Build history of the part. All positions in model axes, mm. Face numbers are marked on the shaded views. A direction names the side the tool comes from. Give positions to 0.01 mm unless a question says otherwise; leave off trailing zeros. Write each loop counter-clockwise with the first axis right and the second up, starting at its lowest first coordinate (ties: lowest second). Pieces come first, ordered by that corner, then holes. Notation, with made-up numbers: (-36, 18.25) -> (13, 18.25) arc R35 cw to (13, 53.25) -> close; hole circle Ø10 at (50.25, 41). An arc over 180 degrees is marked (long way). Write item = value, one per line. Start each with the question number.
Q1. Mould opens along Y. For the marked faces 1, 2 and 3 say: pulls with the +Y half, pulls with the -Y half, needs draft (parallel to the pull), parting line crosses it, or undercut.
Q2. Saw through at B-B, the plane z = 19.5. List the corners of the cut face in (x, y), then the cut area to 3 significant figures.
Q3. Tool access for the marked faces 4, 5, 6, 7 and 8: list every direction of +Z, -Z, +X, -X, +Y, -Y with a clear straight run to the whole face (end or side of a thin tool).
Q4. Wall check: line 1 (X direction, y = -12, z = -21); line 2 (Y direction, x = 19, z = -1); line 3 (Y direction, x = 28.5, z = 4.5). Give the ranges that are in metal, low to high.
Q5. Drop flat-ended pins along their axis: P1, Ø3, axis at x = 3, y = -22, coming from the +Z side; P2, Ø4, axis at x = 28.5, z = 2, coming from the +Y side; P3, Ø4, axis at x = 23, z = -3, coming from the -Y side. Give the stop position or say it passes through.
Q6. Saw through at C-C, the plane y = -16. List the corners of the cut face in (x, z), then the cut area to 3 significant figures.
Q7. Saw through at D-D, the plane x = 13. List the corners of the cut face in (y, z), then the cut area to 3 significant figures.
Q8. Saw through at A-A, the plane z = 0. List the corners of the cut face in (x, y), then the cut area to 3 significant figures.
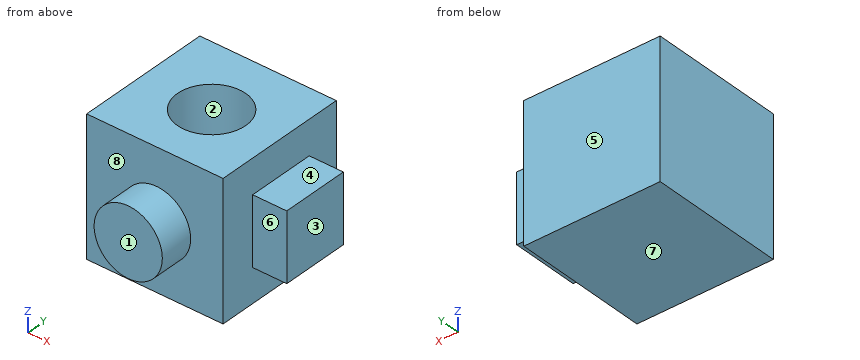
from build123d import *

# Parameters (mm, degrees)
F0_W     = 50.8
F0_H     = 50.8
F1_DEPTH = 50.8
F2_R     = 12.7
F3_DEPTH = 12.7
F4_W     = 25.4
F4_H     = 25.4
F5_DEPTH = 12.7
F6_R     = 12.7
F7_DEPTH = 19.812


with BuildPart() as f1:
    # F0 (on Front) → F1 (new body)
    with BuildSketch(Plane.XZ):
        with Locations((-6.018102, 1.05328)):
            Rectangle(F0_W, F0_H)
    extrude(amount=F1_DEPTH)

    # F2 (on face) → F3 (join)
    with BuildSketch(Plane.XZ.offset(50.8)):
        with Locations((-5.397914, 0)):
            Circle(F2_R)
    extrude(amount=F3_DEPTH)

    # F4 (on face) → F5 (join)
    with BuildSketch(Plane.YZ.offset(19.381898)):
        with Locations((-24.825621, 0.956289)):
            Rectangle(F4_W, F4_H)
    extrude(amount=F5_DEPTH)

    # F6 (on face) → F7 (cut)
    with BuildSketch(Plane.XY.offset(26.45328)):
        with Locations((-5.251253, -26.256265)):
            Circle(F6_R)
    extrude(amount=-F7_DEPTH, mode=Mode.SUBTRACT)


solid = f1.part
Report:
q1.face_1 = pulls with the -Y half
q1.face_2 = undercut
q1.face_3 = needs draft
q2.outline = (-31.42, -50.8) -> (19.38, -50.8) -> (19.38, 0) -> (-31.42, 0) -> close; hole circle Ø25.4 at (-5.25, -26.26)
q2.area = 2,070 mm2
q3.face_4 = +Z, +X, +Y, -Y
q3.face_5 = +Z, -Z, +X, -X, +Y
q3.face_6 = +Z, -Z, +X, -Y
q3.face_7 = -Z, +X, -X, +Y, -Y
q3.face_8 = -Y
q4.line_1 = -31.42 to 19.38
q4.line_2 = -50.8 to 0
q4.line_3 = -37.53 to -12.13
q5.P1 = 6.64
q5.P2 = -12.13
q5.P3 = -37.53
q6.outline = (-31.42, -24.35) -> (19.38, -24.35) -> (19.38, -11.74) -> (32.08, -11.74) -> (32.08, 13.66) -> (19.38, 13.66) -> (19.38, 26.45) -> (2.24, 26.45) -> (2.24, 6.64) -> (-12.74, 6.64) -> (-12.74, 26.45) -> (-31.42, 26.45) -> close
q6.area = 2,610 mm2
q7.outline = (-50.8, -24.35) -> (0, -24.35) -> (0, 26.45) -> (-50.8, 26.45) -> close
q7.area = 2,580 mm2
q8.outline = (-31.42, -50.8) -> (-18.1, -50.8) -> (-18.1, -63.5) -> (7.3, -63.5) -> (7.3, -50.8) -> (19.38, -50.8) -> (19.38, -37.53) -> (32.08, -37.53) -> (32.08, -12.13) -> (19.38, -12.13) -> (19.38, 0) -> (-31.42, 0) -> close
q8.area = 3,230 mm2
